Can you work these out from the drawing? Everything is in mm from the part's minimum corner. Round coordinates to 2 decimals unless told otherwise and drop trailing zeros. Loops run counter-clockwise (first coordinate to the right, second up) from the corner with the lowest first, then second, coordinate; pieces in that order, holes last. Notation, with made-up numbers: (19.5, -34) - (33.5, -34) arc R12 ccw to (33.5, -18) - close; hole circle Ø8 at (15.25, 64.5). An arc over 180 degrees is marked (long way). Answer as CSV lines item,"result". Start each with the question number.
1) Please list where these lines run through material, in increasing order: line 1 along Y through (x, z) = (10, 7.75); line 2 along Z through (x, y) = (10, 28.5); line 3 along X through (y, z) = (27, 4.75).
2) Suppose I cut it at B-B, the plane x = 3. Write out the boundary of the cut face in (y, z).
3) Suppose I cut it at D-D, the plane x = 17.75. Write out the boundary of the cut face in (y, z), then the cut area to 3 significant figures.
4) Suppose I cut it at C-C, the plane z = 8.5. Write out the boundary of the cut face in (x, y), then the cut area to 3 significant figures.
5) We'd pull the mould along X, two halves only. Please class the marked faces 1, 2 and 3: pulls with the +X half, pulls with the -X half, needs draft (parallel to the pull), parting line crosses it, or undercut.
6) I'm going to push a flat-ended pin straight in: pin 1 Ø4 at (x, y) = (10, 22) entering from +Z. Where does the tip first touch, or does it pass through?
7) Suppose I cut it at A-A, the plane x = 10. Write out the boundary of the cut face in (y, z), then the cut area to 3 significant figures.
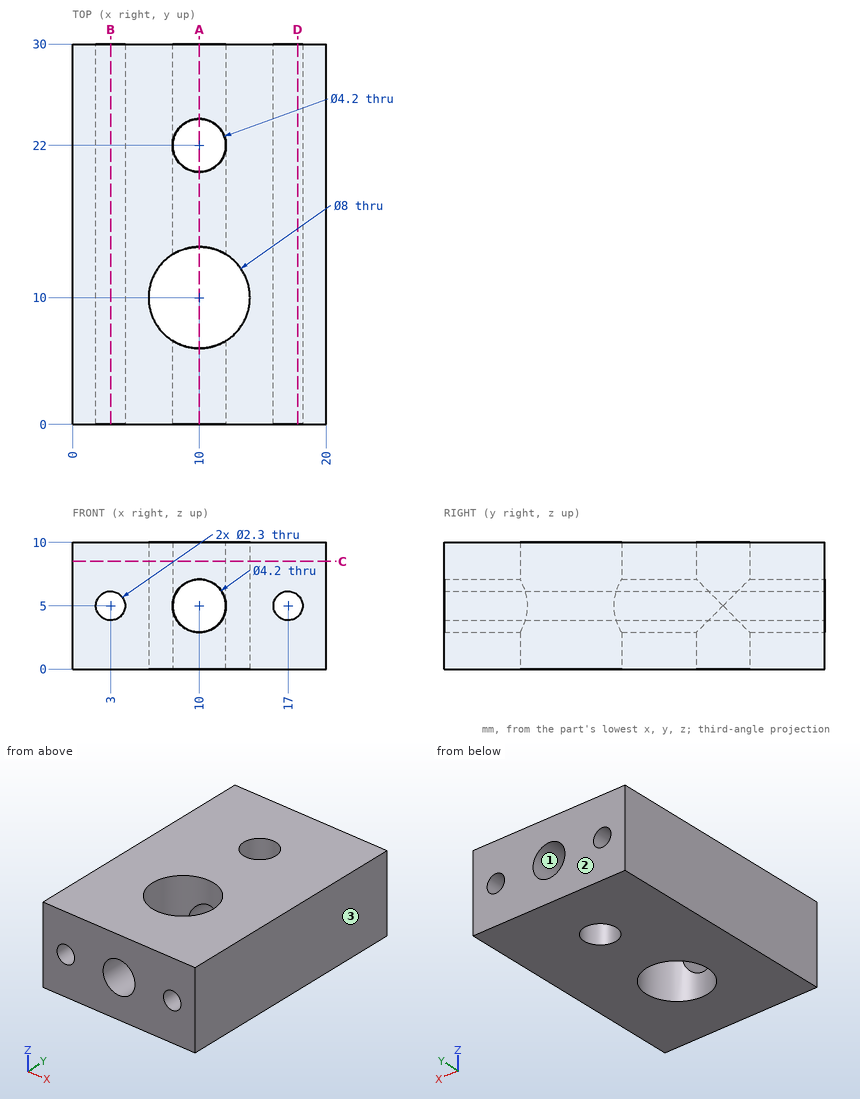
Filled sheet:
1,line 1,"0 to 6, 14 to 19.9, 24.1 to 30"
1,line 2,"0 to 2.9, 7.1 to 10"
1,line 3,"0 to 1.88, 4.12 to 7.91, 12.09 to 15.88, 18.12 to 20"
2,outline,"(0, 0) - (30, 0) - (30, 3.85) - (0, 3.85) - close; (0, 6.15) - (30, 6.15) - (30, 10) - (0, 10) - close"
3,outline,"(0, 0) - (30, 0) - (30, 4.13) - (0, 4.13) - close; (0, 5.87) - (30, 5.87) - (30, 10) - (0, 10) - close"
3,area,"248 mm²"
4,outline,"(0, 0) - (20, 0) - (20, 30) - (0, 30) - close; hole circle Ø8 at (10, 10); hole circle Ø4.2 at (10, 22)"
4,area,"536 mm²"
5,face 1,"undercut"
5,face 2,"needs draft"
5,face 3,"pulls with the +X half"
6,pin 1,"through"
7,outline,"(0, 0) - (6, 0) - (6, 2.9) - (0, 2.9) - close; (0, 7.1) - (6, 7.1) - (6, 10) - (0, 10) - close; (14, 0) - (19.9, 0) - (19.9, 2.9) - (14, 2.9) - close; (14, 7.1) - (19.9, 7.1) - (19.9, 10) - (14, 10) - close; (24.1, 0) - (30, 0) - (30, 2.9) - (24.1, 2.9) - close; (24.1, 7.1) - (30, 7.1) - (30, 10) - (24.1, 10) - close"
7,area,"103 mm²"
